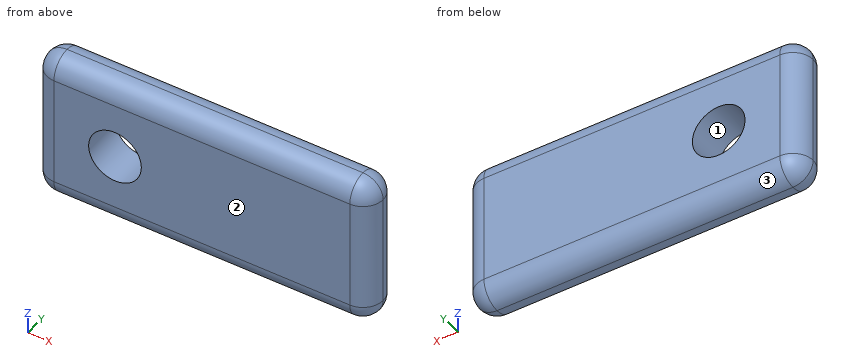
```python
from build123d import *

# Parameters (mm, degrees)
F1_DEPTH = 4.572
F2_R     = 2.28599


# Not quite as in the source:
# - a fillet or chamfer is up to 0.001 mm smaller than in the source, because OpenCascade refuses the exact size


with BuildPart() as f1:
    # F0 (on Front) → F1 (new body)
    with BuildSketch(Plane.XZ):
        with BuildLine():
            Line((-29.10264256, -17.6625937588), (-67.20264256, -17.6625937588))
            Line((-67.20264256, -17.6625937588), (-67.20264256, -26.1715937588))
            Line((-67.20264256, -26.1715937588), (-60.9790929348, -26.1715937588))
            ThreePointArc((-60.9790929348, -26.1715937588), (-57.9945929348, -23.1870937588), (-55.0100929348, -26.1715937588))
            Line((-55.0100929348, -26.1715937588), (-29.10264256, -26.1715937588))
            Line((-29.10264256, -26.1715937588), (-29.10264256, -17.6625937588))
        make_face()
        with BuildLine():
            Line((-60.9790929348, -26.1715937588), (-67.20264256, -26.1715937588))
            Line((-67.20264256, -26.1715937588), (-67.20264256, -34.6805937588))
            Line((-67.20264256, -34.6805937588), (-29.10264256, -34.6805937588))
            Line((-29.10264256, -34.6805937588), (-29.10264256, -26.1715937588))
            Line((-29.10264256, -26.1715937588), (-55.0100929348, -26.1715937588))
            ThreePointArc((-55.0100929348, -26.1715937588), (-57.9945929348, -29.1560937588), (-60.9790929348, -26.1715937588))
        make_face()
    extrude(amount=F1_DEPTH)

    # F2 (radius 2.286 in the source; OpenCascade refuses exactly that, so slightly less here)
    f2_edges = [f1.edges().sort_by_distance(p)[0] for p in [
        (-67.202643, -2.286, -17.662594),
        (-29.102643, -2.286, -17.662594),
        (-29.102643, -2.286, -34.680594),
        (-67.202643, -2.286, -34.680594),
        (-48.152643, -4.572, -34.680594),
        (-48.152643, 0, -34.680594),
        (-29.102643, 0, -26.171594),
        (-29.102643, -4.572, -26.171594),
        (-48.152643, -4.572, -17.662594),
        (-48.152643, 0, -17.662594),
        (-67.202643, 0, -26.171594),
        (-67.202643, -4.572, -26.171594),
    ]]
    fillet(f2_edges, radius=F2_R)


solid = f1.part
```
Geometry check sheet. Reference: the model listing, model coordinates, mm. Face numbers are marked on the shaded views. Round coordinates to 2 decimals unless told otherwise and drop trailing zeros. Write each loop counter-clockwise with the first axis right and the second up, starting at its lowest first coordinate (ties: lowest second). Pieces come first, ordered by that corner, then holes. Notation, with made-up numbers: (-11.75, 27) -> (29.25, 27) arc R22 ccw to (29.25, 33) -> close; hole circle Ø10 at (0, 8). An arc over 180 degrees is marked (long way). Put each result on its own line as item: value.
1) Thickness scan on probe 1 along Z at (x, y) = (-60, -4.05); probe 2 along X at (y, z) = (-2.75, -27.5); probe 3 along X at (y, z) = (-0.95, -24). Record the ranges inside material, lowest first. Write a range as from..to.
Recorded:
probe 1: z = -33.85..-28.38, -23.96..-18.49
probe 2: x = -67.16..-60.67, -55.32..-29.15
probe 3: x = -66.77..-60.04, -55.95..-29.53
2) Depth check by flat-ended pin: P1, Ø1.5, axis at x = -56, y = -4, coming from the -Z side; P2, Ø1.5, axis at y = -4, z = -26, coming from the -X side. Enter the tip coordinate at first touch or a pass-through.
Recorded:
P1: stops at z = -34.47
P2: stops at x = -66.99
3) Cross-section at C-C, the plane y = -1.55. Enter the section's corners in (x, z).
Recorded:
outline: (-67.08, -32.39) arc R2.16 ccw to (-64.92, -34.56) -> (-31.39, -34.56) arc R2.16 ccw to (-29.22, -32.39) -> (-29.22, -19.95) arc R2.16 ccw to (-31.39, -17.78) -> (-64.92, -17.78) arc R2.16 ccw to (-67.08, -19.95) -> close; hole circle Ø5.97 at (-57.99, -26.17)
4) Release check for a two-part mould opening along Y. For the marked faces 1, 2 and 3 record: pulls with the +Y half, pulls with the -Y half, needs draft (parallel to the pull), parting line crosses it, or undercut.
Recorded:
face 1: needs draft
face 2: pulls with the -Y half
face 3: pulls with the +Y half
